```python
from build123d import *

# Parameters (mm, degrees)
SKETCH1_R           = 60
BOSS_EXTRUDE1_DEPTH = 120
BOSS_EXTRUDE2_DEPTH = 30
CUT_EXTRUDE1_REACH  = 154.263
SKETCH3_W           = 6
SKETCH3_H           = 6
SKETCH4_R           = 4
CUT_EXTRUDE2_DEPTH  = 30


with BuildPart() as part:
    # Sketch1 → Boss-Extrude1 (new body)
    with BuildSketch(Plane(origin=(0, 0, 0), x_dir=(1, 0, 0), z_dir=(0, 1, 0))):
        with Locations(Location((0, 0, 0), (0, 0, 270))):
            Circle(SKETCH1_R)
    extrude(amount=-BOSS_EXTRUDE1_DEPTH)

    # Sketch2 → Boss-Extrude2 (add)
    with BuildSketch(Plane(origin=(0, 0, 0), x_dir=(1, 0, 0), z_dir=(0, 1, 0))):
        with BuildLine():
            Line((-12, 9), (-12, -9))
            ThreePointArc((-12, -9), (0, -15), (12, -9))
            Line((12, -9), (12, 9))
            ThreePointArc((12, 9), (0, 15), (-12, 9))
        make_face()
    extrude(amount=BOSS_EXTRUDE2_DEPTH)

    # Sketch3 → Cut-Extrude1 (cut, up to next)
    with BuildSketch(Plane(origin=(12, 0, 0), x_dir=(0, 0, -1), z_dir=(1, 0, 0)), mode=Mode.PRIVATE) as cut_extrude1_sk1:
        with Locations((-12, 18)):
            Rectangle(SKETCH3_W, SKETCH3_H)
    cut_extrude1_tool1 = extrude(cut_extrude1_sk1.sketch, amount=-CUT_EXTRUDE1_REACH, mode=Mode.PRIVATE) & part.part
    cut_extrude1 = cut_extrude1_tool1.solids().sort_by_distance((12, 18, 12))[0]
    add(cut_extrude1, mode=Mode.SUBTRACT)

    # Mirror1: Cut-Extrude1 across plane
    add(cut_extrude1.mirror(Plane.XY), mode=Mode.SUBTRACT)

    # Sketch4 → Cut-Extrude2 (cut)
    with BuildSketch(Plane(origin=(0, 30, 0), x_dir=(1, 0, 0), z_dir=(0, 1, 0))):
        with Locations(Location((0, 0, 0), (0, 0, 270))):
            Circle(SKETCH4_R)
    extrude(amount=-CUT_EXTRUDE2_DEPTH, mode=Mode.SUBTRACT)


solid = part.part
```
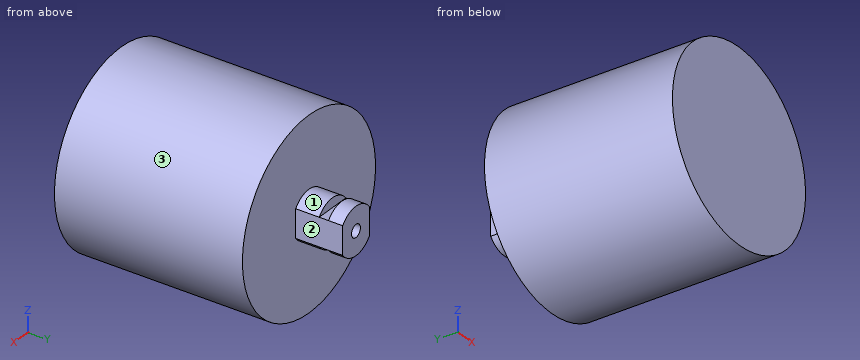
Work out the finished part from the listing and answer in its coordinate system (mm). Face numbers are marked on the shaded views. A direction names the side the tool comes from. Coordinates: 2 decimals unless noted, no trailing zeros. Loops run counter-clockwise (first coordinate to the right, second up) from the corner with the lowest first, then second, coordinate; pieces in that order, holes last.
1) Section A-A (z = 0) is taken. Give the vertices of the cut face in (x, y).
Results:
outline: (-60, -120) - (60, -120) - (60, 0) - (12, 0) - (12, 30) - (4, 30) - (4, 0) - (-4, 0) - (-4, 30) - (-12, 30) - (-12, 0) - (-60, 0) - close
2) Section B-B (y = 19) is taken. Give the vertices of the cut face in (x, z).
Results:
outline: (-12, -9) - (12, -9) - (12, 9) - (-12, 9) - close; hole circle Ø8 at (0, 0)
3) Flat-ended cylindrical pins translate along their axes: pin 1 (1.8 mm diameter, centred on x = 0.5, y = 19, fed in from +Z); pin 2 (2 mm diameter, centred on x = 4, y = -23, fed in from -Z); pin 3 (20 mm diameter, centred on y = 12, z = 2, fed in from +X); pin 4 (8 mm diameter, centred on y = 7.5, z = -46, fed in from -X). Find the tip coordinate at first contact, or state that the pin passes through.
Results:
pin 1: stops at z = 9
pin 2: stops at z = -59.92
pin 3: stops at x = 12
pin 4: passes through
4) Section D-D (y = -81) is taken. Give the vertices of the cut face in (x, z).
Results:
outline: circle Ø120 at (0, 0)
5) Section C-C (x = 0) is taken. Give the vertices of the cut face in (y, z).
Results:
outline: (-120, -60) - (0, -60) - (0, -15) - (15, -15) - (15, -9) - (21, -9) - (21, -15) - (30, -15) - (30, -4) - (0, -4) - (0, 4) - (30, 4) - (30, 15) - (21, 15) - (21, 9) - (15, 9) - (15, 15) - (0, 15) - (0, 60) - (-120, 60) - close
6) Consider probe 1 along X at (y, z) = (14, 0); probe 2 along X at (y, z) = (-88.5, -1); probe 3 along Y at (x, z) = (-27.5, -36). Determine where each line is inside the solid, lowest interval first.
Results:
probe 1: x = -12 to -4, 4 to 12
probe 2: x = -59.99 to 59.99
probe 3: y = -120 to 0
7) For the marked faces 1, 2 and 3, determine the directions among +Z, -Z, +X, -X, +Y, -Y from which every point of the face is accessible in a straight line to the end or side of a thin tool.
Results:
face 1: +Z, +Y
face 2: +Z, -Z, +X, +Y
face 3: +Y, -Y
